```python
from build123d import *

# Parameters (mm, degrees)
SKETCH1_W           = 254
SKETCH1_H           = 181.61
BOSS_EXTRUDE1_DEPTH = 5.08
SKETCH2_R           = 15.875
CUT_EXTRUDE1_DEPTH  = 5.08
SKETCH3_R           = 1.5875
CUT_EXTRUDE3_DEPTH  = 7.62
SKETCH5_R           = 2.794
CUT_EXTRUDE5_DEPTH  = 3.302
SKETCH6_R           = 1.5875
CUT_EXTRUDE6_DEPTH  = 5.08


with BuildPart() as part:
    # Sketch1 → Boss-Extrude1 (new body)
    with BuildSketch(Plane.XY):
        with Locations((127, 90.805)):
            Rectangle(SKETCH1_W, SKETCH1_H)
    extrude(amount=BOSS_EXTRUDE1_DEPTH)

    # Sketch2 → Cut-Extrude1 (cut)
    with BuildSketch(Plane.XY.offset(5.08)):
        with Locations((127, 90.805)):
            Circle(SKETCH2_R)
    extrude(amount=-CUT_EXTRUDE1_DEPTH, mode=Mode.SUBTRACT)

    # Sketch3 → Cut-Extrude3 (cut)
    with BuildSketch(Plane.XY.offset(5.08)):
        with Locations((7.62, 173.99)):
            Circle(SKETCH3_R)
        with Locations((246.38, 173.99)):
            Circle(SKETCH3_R)
        with Locations((7.62, 7.62)):
            Circle(SKETCH3_R)
        with Locations((246.38, 7.62)):
            Circle(SKETCH3_R)
    extrude(amount=-CUT_EXTRUDE3_DEPTH, mode=Mode.SUBTRACT)

    # Sketch5 → Cut-Extrude5 (cut)
    with BuildSketch(Plane.XY.offset(5.08)):
        with Locations((246.38, 173.99)):
            Circle(SKETCH5_R)
        with Locations((246.38, 7.62)):
            Circle(SKETCH5_R)
        with Locations((7.62, 173.99)):
            Circle(SKETCH5_R)
        with Locations((7.62, 7.62)):
            Circle(SKETCH5_R)
    extrude(amount=-CUT_EXTRUDE5_DEPTH, mode=Mode.SUBTRACT)

    # Sketch6 → Cut-Extrude6 (cut)
    with BuildSketch(Plane.XY.offset(5.08)):
        with Locations((127, 147.955)):
            Circle(SKETCH6_R)
        with Locations((184.15, 90.805)):
            Circle(SKETCH6_R)
        with Locations((127, 33.655)):
            Circle(SKETCH6_R)
        with Locations((69.85, 90.805)):
            Circle(SKETCH6_R)
        with Locations((163.83, 90.805)):
            Circle(SKETCH6_R)
        with Locations((127, 53.848)):
            Circle(SKETCH6_R)
        with Locations((90.043, 90.805)):
            Circle(SKETCH6_R)
        with Locations((126.746, 127.761127137)):
            Circle(SKETCH6_R)
    extrude(amount=-CUT_EXTRUDE6_DEPTH, mode=Mode.SUBTRACT)


solid = part.part
```
Part model, mm, in its own coordinate system. A direction names the side the tool comes from. Coordinates: 2 decimals unless noted, no trailing zeros. Order: outer loops, then holes, each group sorted by start corner. A loop starts at its lowest first (then second) coordinate and runs counter-clockwise, first axis right, second up. Notation, with made-up numbers: (-31.75, 26.5) -> (-18.75, 26.5) arc R26 ccw to (-18.75, 48.5) -> close; hole circle Ø2 at (58, 72.25). An arc over 180 degrees is marked (long way). Put each result on its own line as item: value. Start each with the question number.
(1) Band-saw the part on B-B (x = 134.5). Give the cut face in (y, z), then the cut area to 3 significant figures.
(2) Probe line 1 along X through (y, z) = (173.99, 1); line 2 along Y through (x, z) = (7.62, 2.45); line 3 along Y through (x, z) = (127, 1.4). List the from-to ranges inside material, lowest first. Write a range as [from, to].
(3) Mould opens along Y. For faces 3 (the face through (254, 90, 3)), 4 (the face through (248, 173, 1.778)), 5 (the face through (125, 0, 3)) say: pulls with the +Y half, pulls with the -Y half, needs draft (parallel to the pull), parting line crosses it, or undercut.
(4) Band-saw the part on C-C (y = 96). Give the cut face in (x, z), then the cut area to 3 significant figures.
(5) Band-saw the part on A-A (z = 4.05). Count the separate pieces of the cut face and the enclosed holes in it, then the cut area to 3 significant figures.
(6) Which spindle directions (+Z, -Z, +X, -X, +Y, -Y) get a long thin tool onto all of the face, cutting with end or side? Do faces 1 (the face through (249.045, 8.459, 3.452)), 2 (the face through (114.4, 81.15, 2.58)). Say none if no direction does.
(7) Pin check, flat tips, straight feed: pin 1 Ø1.9 at (x, y) = (127, 53.848) entering from -Z; pin 2 Ø4 at (x, y) = (7.62, 173.99) entering from +Z. Stop position of each tip, or through.
Determined:
1. outline: (0, 0) -> (76.81, 0) -> (76.81, 5.08) -> (0, 5.08) -> close; (104.8, 0) -> (181.61, 0) -> (181.61, 5.08) -> (104.8, 5.08) -> close
1. area: 780 mm²
2. line 1: x = [0, 6.03], [9.21, 244.79], [247.97, 254]
2. line 2: y = [0, 4.83], [10.41, 171.2], [176.78, 181.61]
2. line 3: y = [0, 32.07], [35.24, 52.26], [55.44, 74.93], [106.68, 126.19], [129.33, 146.37], [149.54, 181.61]
3. face 3: needs draft
3. face 4: undercut
3. face 5: pulls with the -Y half
4. outline: (0, 0) -> (112, 0) -> (112, 5.08) -> (0, 5.08) -> close; (142, 0) -> (254, 0) -> (254, 5.08) -> (142, 5.08) -> close
4. area: 1,140 mm²
5. separate pieces: 1
5. enclosed holes: 13
5. area: 45,200 mm²
6. face 1: +Z
6. face 2: +Z, -Z
7. pin 1: passes through
7. pin 2: stops at z = 1.78
